Source: three-view drawing plus pictorial views. Frame: mm from the lowest corner of the part. Give positions to 0.01 mm unless a question says otherwise; leave off trailing zeros. Loops run counter-clockwise (first coordinate to the right, second up) from the corner with the lowest first, then second, coordinate; pieces in that order, holes last.
1. Material intervals for line 1 along X through (y, z) = (33.5, 52); line 2 along X through (y, z) = (34, 6); line 3 along X through (y, z) = (16, 80), sorted ascending.
2. Section A-A, the plane y = 31. Output: boundary loops of the cut face in (x, z).
3. Section B-B, the plane z = 26. Output: boundary loops of the cut face in (x, y) (1 decimal), then the cut area to 3 significant figures.
4. Draft query along X for the marked faces 1 and 2. Return one class per face: +X half, -X half, draft (parallel to the pull), parting line (faces both ways), or undercut.
5. First-contact query: P1, Ø21, axis at y = 31.5, z = 43.5, coming from the -X side; P2, Ø19, axis at y = 11, z = 75, coming from the -X side; P3, Ø21, axis at x = 499.5, z = 39, coming from the +Y side (1 decimal); P4, Ø19, axis at x = 42.5, y = 16, coming from the +Z side. Flat tips, straight axial feed; report the tip coordinate or a pass-through.
6. Section C-C, the plane x = 76.5. Output: boundary loops of the cut face in (y, z), then the cut area to 3 significant figures.
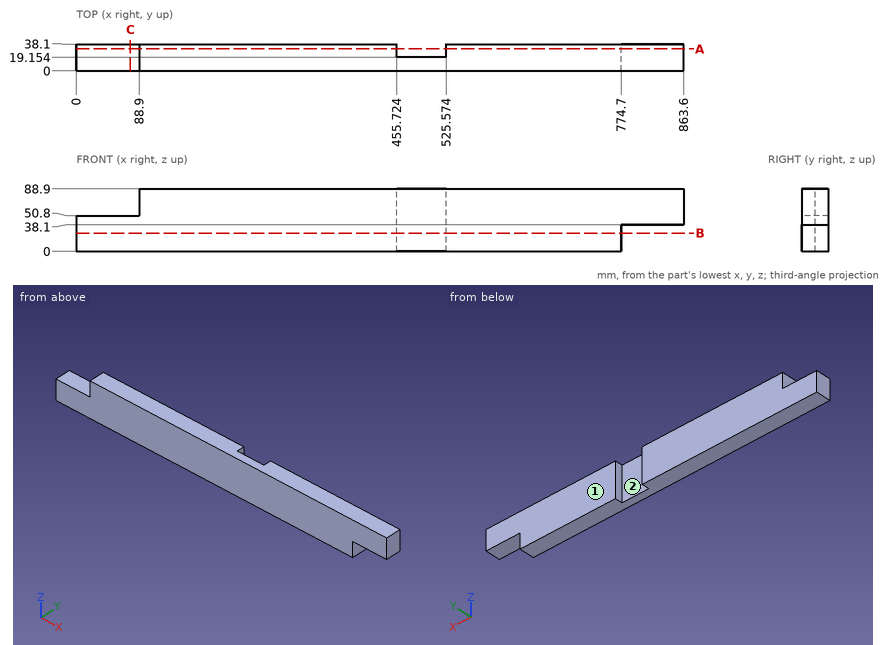
Answers below:
1. line 1: x = 88.9 to 455.72, 525.57 to 863.6
1. line 2: x = 0 to 455.72, 525.57 to 774.7
1. line 3: x = 88.9 to 863.6
2. outline: (0, 0) - (455.72, 0) - (455.72, 88.9) - (88.9, 88.9) - (88.9, 50.8) - (0, 50.8) - close; (525.57, 0) - (774.7, 0) - (774.7, 38.1) - (863.6, 38.1) - (863.6, 88.9) - (525.57, 88.9) - close
3. outline: (0, 0) - (774.7, 0) - (774.7, 38.1) - (525.6, 38.1) - (525.6, 19.2) - (455.7, 19.2) - (455.7, 38.1) - (0, 38.1) - close
3. area: 28,200 mm2
4. face 1: draft
4. face 2: undercut
5. P1: stops at x = 0
5. P2: stops at x = 88.9
5. P3: stops at y = 19.2
5. P4: stops at z = 50.8
6. outline: (0, 0) - (38.1, 0) - (38.1, 50.8) - (0, 50.8) - close
6. area: 1,940 mm2
